CAD build for the part. Positions are in the model's coordinates, mm. A direction names the side the tool comes from. Coordinates: 2 decimals unless noted, no trailing zeros. Order: outer loops, then holes, each group sorted by start corner. A loop starts at its lowest first (then second) coordinate and runs counter-clockwise, first axis right, second up. Notation, with made-up numbers: (66.5, 44.25) - (74.5, 44.25) arc R23 cw to (74.5, 63.25) - close; hole circle Ø2 at (4, 68). An arc over 180 degrees is marked (long way). Return JSON: item names as keys, results as strings.
from build123d import *

# Parameters (mm, degrees)
SKETCH_1_W      = 23.2
SKETCH_1_H      = 22.7
SKETCH_1_R      = 1.65
EXTRUDE_1_DEPTH = 3
FILLET_1_R      = 3
SKETCH_2_W      = 4.543947028
SKETCH_2_H      = 5.301271532
EXTRUDE_2_DEPTH = 1


with BuildPart() as part:
    # 草图1 → 凸台-拉伸1 (new body)
    with BuildSketch(Plane(origin=(0, 0, 0), x_dir=(1, 0, 0), z_dir=(0, 1, 0))):
        Rectangle(SKETCH_1_W, SKETCH_1_H)
        with Locations(Location((-8, 8, 0), (0, 0, 270))):
            Circle(SKETCH_1_R, mode=Mode.SUBTRACT)
        with Locations(Location((8, 8, 0), (0, 0, 270))):
            Circle(SKETCH_1_R, mode=Mode.SUBTRACT)
        with Locations(Location((8, -8, 0), (0, 0, 270))):
            Circle(SKETCH_1_R, mode=Mode.SUBTRACT)
        with Locations(Location((-8, -8, 0), (0, 0, 270))):
            Circle(SKETCH_1_R, mode=Mode.SUBTRACT)
    extrude(amount=EXTRUDE_1_DEPTH)

    # 圆角1
    fillet_1_edges = [part.edges().sort_by_distance(p)[0] for p in [
        (11.6, 1.5, 11.35),
        (-11.6, 1.5, 11.35),
        (-11.6, 1.5, -11.35),
        (11.6, 1.5, -11.35),
    ]]
    fillet(fillet_1_edges, radius=FILLET_1_R)

    # 草图2 → 凸台-拉伸2 (add)
    with BuildSketch(Plane(origin=(0, 3, 0), x_dir=(1, 0, 0), z_dir=(0, 1, 0))):
        Rectangle(SKETCH_2_W, SKETCH_2_H)
    extrude(amount=EXTRUDE_2_DEPTH)


solid = part.part
Item 1: Wall check: L1, parallel to X at y = 0.95, z = 8; L2, parallel to X at y = 1.85, z = 6.5; L3, parallel to Z at x = -8.5, y = 1.05. Give the ranges that are in metal, low to high. Write a range as [from, to].
Findings below:
{"L1": "x = [-11.6, -9.65], [-6.35, 6.35], [9.65, 11.6]", "L2": "x = [-11.6, -8.69], [-7.31, 7.31], [8.69, 11.6]", "L3": "z = [-11.35, -9.57], [-6.43, 6.43], [9.57, 11.35]"}
Item 2: Mould opens along X. For faces 4 (the flat face through (0, 3.5, -2.651)), 5 (the cylindrical face through (9.115, 1.479, 6.784)), 6 (the flat face through (2.272, 3.5, 0)) say: released by +X, released by -X, zero draft, split by the parting line, or undercut.
Findings below:
{"face 4": "zero draft", "face 5": "undercut", "face 6": "released by +X"}
Item 3: Which spindle directions (+Z, -Z, +X, -X, +Y, -Y) get a long thin tool onto all of the face, cutting with end or side? Do faces 1 (the flat face through (-2.272, 3.5, 0)), 2 (the flat face through (0, 3.5, 2.651)), 3 (the cylindrical face through (-6.885, 1.479, 6.784)). Say none if no direction does.
Findings below:
{"face 1": "+Z, -Z, -X, +Y", "face 2": "+Z, +X, -X, +Y", "face 3": "+Y, -Y"}
Item 4: Drop flat-ended pins along their axis: P1, Ø6, axis at x = 5.5, z = -8, coming from the +Y side; P2, Ø0.5, axis at x = 0, y = 3.5, coming from the +Z side; P3, Ø0.5, axis at x = 0.5, y = 3.5, coming from the -Z side. Give the stop position or say it passes through.
Findings below:
{"P1": "stops at y = 3", "P2": "stops at z = 2.65", "P3": "stops at z = -2.65"}
Item 5: Band-saw the part on C-C, the plane z = -2. List the corners of the cut face in (x, y), then the cut area to 3 significant figures.
Findings below:
{"outline": "(-11.6, 0) - (11.6, 0) - (11.6, 3) - (2.27, 3) - (2.27, 4) - (-2.27, 4) - (-2.27, 3) - (-11.6, 3) - close", "area": "74.1 mm²"}
Item 6: Band-saw the part on D-D, the plane z = 8. List the corners of the cut face in (x, y), then the cut area to 3 significant figures.
Findings below:
{"outline": "(-11.6, 0) - (-9.65, 0) - (-9.65, 3) - (-11.6, 3) - close; (-6.35, 0) - (6.35, 0) - (6.35, 3) - (-6.35, 3) - close; (9.65, 0) - (11.6, 0) - (11.6, 3) - (9.65, 3) - close", "area": "49.8 mm²"}
Item 7: Band-saw the part on A-A, the plane x = -8. List the corners of the cut face in (y, z).
Findings below:
{"outline": "(0, -11.35) - (3, -11.35) - (3, -9.65) - (0, -9.65) - close; (0, -6.35) - (3, -6.35) - (3, 6.35) - (0, 6.35) - close; (0, 9.65) - (3, 9.65) - (3, 11.35) - (0, 11.35) - close"}
Item 8: Band-saw the part on B-B, the plane y = 2.05. List the corners of the cut face in (x, z), then the cut area to 3 significant figures.
Findings below:
{"outline": "(-11.6, -8.35) arc R3 ccw to (-8.6, -11.35) - (8.6, -11.35) arc R3 ccw to (11.6, -8.35) - (11.6, 8.35) arc R3 ccw to (8.6, 11.35) - (-8.6, 11.35) arc R3 ccw to (-11.6, 8.35) - close; hole circle Ø3.3 at (-8, -8); hole circle Ø3.3 at (-8, 8); hole circle Ø3.3 at (8, -8); hole circle Ø3.3 at (8, 8)", "area": "485 mm²"}
